Geometry: final body of the model. Coordinates: model frame, mm. A direction names the side the tool comes from. Round coordinates to 2 decimals unless told otherwise and drop trailing zeros. Loops run counter-clockwise (first coordinate to the right, second up) from the corner with the lowest first, then second, coordinate; pieces in that order, holes last. Notation, with made-up numbers: M -9,32 L 43,32 A17 ccw 43,47 Z; hole C 53,14.25 d6. An arc over 180 degrees is marked long. Answer as a JSON object with one key per item and string values.
from build123d import *

# Parameters (mm, degrees)
SKETCH_1_W                    = 38
SKETCH_1_H                    = 94
EXTRUDE_604_DEPTH             = 6
CUT_EXTRUDE_1_DEPTH           = 78.601546376
CUT_EXTRUDE_1_DEPTH_BACK      = 78.601546376
SKETCH_5_R                    = 5
SKETCH_8_R                    = 27
EXTRUDE_996_DEPTH             = 5
EXTRUDE_996_DIRECTION_2_REACH = 79.602
SKETCH_6_R                    = 1.75
CUT_EXTRUDE_1278_DEPTH        = 81.467384697
SKETCH_16_R                   = 16.175
CUT_EXTRUDE_1486_DEPTH        = 7
SKETCH_7_R                    = 4.5
SKETCH_7_R_2                  = 7.5
CUT_EXTRUDE_1931_DEPTH        = 3
SKETCH_10_R                   = 3.5
CUT_EXTRUDE_2130_DEPTH        = 5
SKETCH_11_R                   = 1.65
CUT_EXTRUDE_2456_DEPTH        = 81.467384697
CUT_EXTRUDE_3_DEPTH           = 5
CHAMFER_1_SIZE                = 1.5
FILLET_5_R                    = 4
SKETCH_17_R                   = 7
CUT_EXTRUDE_3397_DEPTH        = 81.018747803
EXTRUDE_START                 = 0.5
SKETCH_18_R                   = 16.175
SKETCH_18_R_2                 = 15.5
EXTRUDE_3543_DEPTH            = 0.5
SKETCH_19_R                   = 1
CUT_EXTRUDE_3835_DEPTH        = 89.667919791
FILLET_6_R                    = 3


with BuildPart() as part:
    # Эскиз1 → Extrude 604 (new body)
    with BuildSketch(Plane.XY):
        with Locations((0, 28)):
            Rectangle(SKETCH_1_W, SKETCH_1_H)
    extrude(amount=EXTRUDE_604_DEPTH)

    # Эскиз5 → ось двигателя1 (cut, two sides: drawn at the far end of the back side and taken through both)
    with BuildSketch(Plane.XY.offset(6).offset(-CUT_EXTRUDE_1_DEPTH_BACK)):
        Circle(SKETCH_5_R)
    extrude(amount=CUT_EXTRUDE_1_DEPTH + CUT_EXTRUDE_1_DEPTH_BACK, mode=Mode.SUBTRACT)

    # Эскиз8 → Extrude 996 (add)
    with BuildSketch(Plane.XY.offset(6)):
        Circle(SKETCH_8_R)
    extrude(amount=EXTRUDE_996_DEPTH)

    # Extrude 996 direction 2: up to this face of the body (flat: up to its plane)
    extrude_996_direction_2_end = Plane(part.part.faces().sort_by_distance((0, 28.629494754, 0))[0])
    # Эскиз8 → Extrude 996 direction 2 (add, up to the picked face)
    with BuildSketch(Plane.XY.offset(6), mode=Mode.PRIVATE) as extrude_996_direction_2_sk1:
        Circle(SKETCH_8_R)
    extrude_996_direction_2_tool1 = split(extrude(extrude_996_direction_2_sk1.sketch, amount=-EXTRUDE_996_DIRECTION_2_REACH, mode=Mode.PRIVATE), bisect_by=extrude_996_direction_2_end, keep=Keep.BOTH, mode=Mode.PRIVATE)
    add(extrude_996_direction_2_tool1.solids().sort_by(Axis((0, 0, 6), (0, 0, -1)))[0])

    # Эскиз6 → Cut-Extrude 1278 (cut, through all)
    with BuildSketch(Plane(origin=(0, 0, 0), x_dir=(-1, 0, 0), z_dir=(0, 0, -1))):
        with Locations((-9, 24)):
            Circle(SKETCH_6_R)
        with Locations((9, 24)):
            Circle(SKETCH_6_R)
        with Locations((9, -9)):
            Circle(SKETCH_6_R)
        with Locations((-9, -9)):
            Circle(SKETCH_6_R)
    extrude(amount=-CUT_EXTRUDE_1278_DEPTH, mode=Mode.SUBTRACT)

    # Эскиз16 → Cut-Extrude 1486 (cut)
    with BuildSketch(Plane.XY.offset(11)):
        Circle(SKETCH_16_R)
    extrude(amount=-CUT_EXTRUDE_1486_DEPTH, mode=Mode.SUBTRACT)

    # Эскиз7 → Cut-Extrude 1931 (cut)
    with BuildSketch(Plane(origin=(0, 0, 0), x_dir=(-1, 0, 0), z_dir=(0, 0, -1))):
        with Locations((-9, 24)):
            Circle(SKETCH_7_R)
        with Locations((9, 24)):
            Circle(SKETCH_7_R)
        with Locations((-9, -9)):
            Circle(SKETCH_7_R)
        with Locations((9, -9)):
            Circle(SKETCH_7_R)
        Circle(SKETCH_7_R_2)
        with BuildLine():
            Line((-5, 16.5), (5, 16.5))
            ThreePointArc((5, 16.5), (8.5, 13), (5, 9.5))
            Line((5, 9.5), (-5, 9.5))
            ThreePointArc((-5, 9.5), (-8.5, 13), (-5, 16.5))
        make_face()
    extrude(amount=-CUT_EXTRUDE_1931_DEPTH, mode=Mode.SUBTRACT)

    # Эскиз10 → Cut-Extrude 2130 (cut)
    with BuildSketch(Plane.XY.offset(11)):
        with Locations((-9, 24)):
            Circle(SKETCH_10_R)
        with Locations((9, 24)):
            Circle(SKETCH_10_R)
    extrude(amount=-CUT_EXTRUDE_2130_DEPTH, mode=Mode.SUBTRACT)

    # Эскиз11 → Cut-Extrude 2456 (cut, through all)
    with BuildSketch(Plane.XY.offset(11)):
        with Locations((21, 0)):
            Circle(SKETCH_11_R)
        with Locations((-21, 0)):
            Circle(SKETCH_11_R)
        with Locations((0, -21)):
            Circle(SKETCH_11_R)
    extrude(amount=-CUT_EXTRUDE_2456_DEPTH, mode=Mode.SUBTRACT)

    # Эскиз12 → Вырез-Вытянуть3 (cut)
    with BuildSketch(Plane(origin=(0, 0, 0), x_dir=(-1, 0, 0), z_dir=(0, 0, -1))):
        Polygon((-18.1, 1.674315781), (-21, 3.348631561), (-23.9, 1.674315781), (-23.9, -1.674315781), (-21, -3.348631561), (-18.1, -1.674315781), align=None)
        Polygon((2.9, -19.325684219), (0, -17.651368439), (-2.9, -19.325684219), (-2.9, -22.674315781), (0, -24.348631561), (2.9, -22.674315781), align=None)
        Polygon((23.9, 1.674315781), (21, 3.348631561), (18.1, 1.674315781), (18.1, -1.674315781), (21, -3.348631561), (23.9, -1.674315781), align=None)
    extrude(amount=-CUT_EXTRUDE_3_DEPTH, mode=Mode.SUBTRACT)

    # Фаска1
    # the kernel refuses this chamfer: 1.5 mm, written as the material it takes off along each edge
    with BuildSketch(Plane(origin=(-9, 24, 6), x_dir=(-1, 0, 0), z_dir=(0, -1, 0))) as chamfer_1_piece_1:
        Polygon((1.75 + CHAMFER_1_SIZE, 0), (1.75, CHAMFER_1_SIZE), (1.75, 0), align=None)
    revolve(axis=Axis((-9, 24, 6), (0, 0, -1)), mode=Mode.SUBTRACT)
    with BuildSketch(Plane(origin=(9, -9, 4), x_dir=(-1, 0, 0), z_dir=(0, -1, 0))) as chamfer_1_piece_2:
        Polygon((1.75, CHAMFER_1_SIZE), (1.75 + CHAMFER_1_SIZE, 0), (1.75, 0), align=None)
    revolve(axis=Axis((9, -9, 4), (0, 0, -1)), mode=Mode.SUBTRACT)
    with BuildSketch(Plane(origin=(-9, -9, 4), x_dir=(-1, 0, 0), z_dir=(0, -1, 0))) as chamfer_1_piece_3:
        Polygon((1.75, CHAMFER_1_SIZE), (1.75 + CHAMFER_1_SIZE, 0), (1.75, 0), align=None)
    revolve(axis=Axis((-9, -9, 4), (0, 0, -1)), mode=Mode.SUBTRACT)
    with BuildSketch(Plane(origin=(9, 24, 6), x_dir=(-1, 0, 0), z_dir=(0, -1, 0))) as chamfer_1_piece_4:
        Polygon((1.75 + CHAMFER_1_SIZE, 0), (1.75, CHAMFER_1_SIZE), (1.75, 0), align=None)
    revolve(axis=Axis((9, 24, 6), (0, 0, -1)), mode=Mode.SUBTRACT)

    # Скругление5
    fillet_5_edges = [part.edges().sort_by_distance(p)[0] for p in [
        (-19, 19.183326093, 3),
        (19, 19.183326093, 3),
    ]]
    fillet(fillet_5_edges, radius=FILLET_5_R)

    # Эскиз17 → Cut-Extrude 3397 (cut, through all)
    with BuildSketch(Plane.XY.offset(4)):
        Circle(SKETCH_17_R)
    extrude(amount=-CUT_EXTRUDE_3397_DEPTH, mode=Mode.SUBTRACT)

    # Эскиз18 → Extrude 3543 (add)
    with BuildSketch(Plane.XY.offset(4).offset(EXTRUDE_START)):
        Circle(SKETCH_18_R)
        with Locations(Location((0, 0, 0), (0, 0, 218.075409453))):
            Circle(SKETCH_18_R_2, mode=Mode.SUBTRACT)
    extrude(amount=-EXTRUDE_3543_DEPTH)

    # Эскиз19 → Cut-Extrude 3835 (cut, through all)
    with BuildSketch(Plane(origin=(19, 0, 0), x_dir=(0, 0, -1), z_dir=(1, 0, 0))):
        with Locations(Location((-3, 59.5, 0), (0, 0, 90))):
            Circle(SKETCH_19_R)
        with Locations(Location((-3, 39.5, 0), (0, 0, 90))):
            Circle(SKETCH_19_R)
    extrude(amount=-CUT_EXTRUDE_3835_DEPTH, mode=Mode.SUBTRACT)

    # Скругление6
    fillet_6_edges = [part.edges().sort_by_distance(p)[0] for p in [
        (0, 75, 0),
    ]]
    fillet(fillet_6_edges, radius=FILLET_6_R)


solid = part.part
1) Pin query (flat end, axial travel): P1, Ø2, axis at y = 17.5, z = 2, coming from the +X side; P2, Ø5, axis at y = 36, z = 3, coming from the -X side; P3, Ø3.5, axis at y = 1, z = 2, coming from the -X side. Return the tip coordinate at first contact, or that it passes through.
Results:
{"P1": "x = 21.37", "P2": "x = -19", "P3": "x = -27"}
2) Section query A-A (z = 7.75). Return the cut outline in (x, y) (3 decimals), and give its area (3 significant figures).
Results:
{"outline": "M -12.499,23.933 A27 ccw long 12.499,23.933 A3.5 cw long 6.319,26.25 A27 ccw -6.319,26.25 A3.5 cw long Z; hole C -21,0 d3.3; hole C 0,0 d32.35; hole C 0,-21 d3.3; hole C 21,0 d3.3", "area": "1,390 mm2"}
3) Section query C-C (y = 66). Return the cut outline in (x, z).
Results:
{"outline": "M -19,0 L 19,0 L 19,6 L -19,6 Z"}
4) Ray query, line 1 (Y direction, x = 0, z = 4.3); line 2 (X direction, y = 26, z = 5.5); line 3 (X direction, y = 0, z = 4.25). Return the intervals inside material, ascending.
Results:
{"line 1": "-27 to -24.35, -17.65 to -15.5, 15.5 to 75", "line 2": "-19 to -10.89, -7.11 to 7.11, 10.89 to 19", "line 3": "-27 to -23.9, -18.1 to -15.5, 15.5 to 18.1, 23.9 to 27"}
5) Reachability of faces 5 (the flat face through (11.1, -11.1, 4)), 6 (the cylindrical face through (19.35, 0.07, 8.04)), 7 (the cylindrical face through (-8.5, 13.1, 1.5)), 8 (the flat face through (19, 48, 3)) from +Z, -Z, +X, -X, +Y, -Y: full face, straight path, thin tool, end or side. Return the list, or none.
Results:
{"face 5": "none", "face 6": "+Z, -Z", "face 7": "-Z", "face 8": "+Z, -Z, +X, +Y"}
6) Pull-direction query (X, two-part tool) for faces 1 (the flat face through (0, 75, 4)), 2 (the flat face through (-11.18, -11.07, 4)), 3 (the flat face through (-2.9, -21, 2)), 4 (the cylindrical face through (0, 27, 8)); classes: +X half, -X half, draft (parallel to the pull), parting line (faces both ways), or undercut.
Results:
{"face 1": "draft", "face 2": "undercut", "face 3": "undercut", "face 4": "parting line"}
7) Section query B-B (y = -21). Return the cut outline in (x, z).
Results:
{"outline": "M -16.97,0 L -2.9,0 L -2.9,5 L -1.65,5 L -1.65,11 L -16.97,11 Z; M 1.65,5 L 2.9,5 L 2.9,0 L 16.97,0 L 16.97,11 L 1.65,11 Z"}
